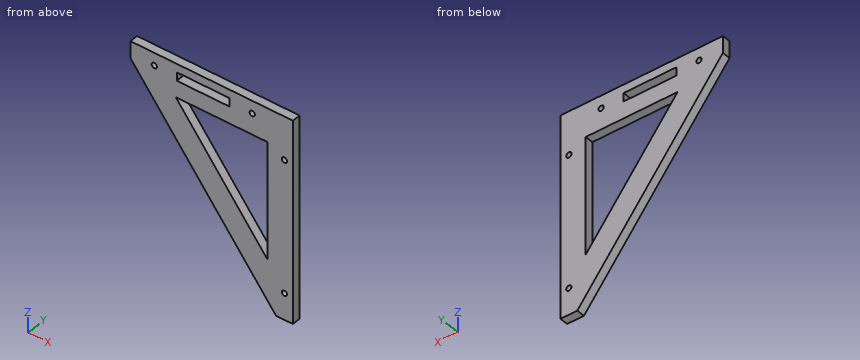
```python
from build123d import *

# Parameters (mm, degrees)
BOSS_EXTRUDE1_DEPTH = 3.175
SKETCH3_W           = 55
SKETCH3_H           = 6.35
BOSS_EXTRUDE3_DEPTH = 3.175
SKETCH5_W           = 6.35
SKETCH5_H           = 76.35
BOSS_EXTRUDE4_DEPTH = 3.175
SKETCH2_R           = 1
SKETCH2_W           = 20
SKETCH2_H           = 3.175
CUT_EXTRUDE1_DEPTH  = 3.175
CUT_EXTRUDE2_DEPTH  = 3.175


with BuildPart() as part:
    # Sketch1 → Boss-Extrude1 (new body)
    with BuildSketch(Plane(origin=(0, 0, 0), x_dir=(1, 0, 0), z_dir=(0, 1, 0))):
        Polygon((0, 0), (55, 0), (55, 70), align=None)
    extrude(amount=BOSS_EXTRUDE1_DEPTH)

    # Sketch3 → Boss-Extrude3 (add)
    with BuildSketch(Plane.XZ):
        with Locations((27.5, 3.175)):
            Rectangle(SKETCH3_W, SKETCH3_H)
    extrude(amount=-BOSS_EXTRUDE3_DEPTH)

    # Sketch5 → Boss-Extrude4 (add)
    with BuildSketch(Plane.XZ):
        with Locations((58.175, -31.825)):
            Rectangle(SKETCH5_W, SKETCH5_H)
    extrude(amount=-BOSS_EXTRUDE4_DEPTH)

    # Sketch2 → Cut-Extrude1 (cut)
    with BuildSketch(Plane(origin=(0, 3.175, 0), x_dir=(1, 0, 0), z_dir=(0, 1, 0))):
        with Locations(Location((9, -1.5875, 0), (0, 0, 270))):
            Circle(SKETCH2_R)
        with Locations(Location((46, -1.5875, 0), (0, 0, 270))):
            Circle(SKETCH2_R)
        with Locations(Location((58.175, 60, 0), (0, 0, 270))):
            Circle(SKETCH2_R)
        with Locations(Location((58.175, 10, 0), (0, 0, 270))):
            Circle(SKETCH2_R)
        with Locations((27.5, -1.5875)):
            Rectangle(SKETCH2_W, SKETCH2_H)
    extrude(amount=-CUT_EXTRUDE1_DEPTH, mode=Mode.SUBTRACT)

    # Sketch6 → Cut-Extrude2 (cut)
    with BuildSketch(Plane(origin=(0, 3.175, 0), x_dir=(1, 0, 0), z_dir=(0, 1, 0))):
        Polygon((51.825, 6.35), (17.102700256, 6.35), (51.825, 50.542017856), align=None)
    extrude(amount=-CUT_EXTRUDE2_DEPTH, mode=Mode.SUBTRACT)


solid = part.part
```
Verification items for the finished model (mm, model axes). Coordinates: 2 decimals unless noted, no trailing zeros. Write each loop counter-clockwise with the first axis right and the second up, starting at its lowest first coordinate (ties: lowest second). Pieces come first, ordered by that corner, then holes. Notation, with made-up numbers: (-16, 31) - (26, 31) arc R22 ccw to (26, 70) - close; hole circle Ø1 at (76.25, 19.25). An arc over 180 degrees is marked (long way). Write item = value, one per line.
Q1. Material ranges on L1, parallel to Z at x = 20, y = 2.9 (3 decimals); L2, parallel to X at y = 1.3, z = -10 (3 decimals); L3, parallel to Z at x = 45.5, y = 2.05, recorded low to high. Write a range as from..to.
Answer:
L1 = -25.455..-10.037, -6.35..0, 3.175..6.35
L2 = 7.857..19.971, 51.825..57.175, 59.175..61.35
L3 = -57.91..-42.49, -6.35..0.72, 2.45..6.35
Q2. Go/stop test with flat-tipped pins: pin 1 Ø1.6 at (x, z) = (46, 1.59) entering from -Y; pin 2 Ø1 at (y, z) = (1.5, -37.5) entering from -X; pin 3 Ø3 at (x, z) = (58.175, -60) entering from -Y. Record where each tip stops, or that it passes through.
Answer:
pin_1 = through
pin_2 = 29.07
pin_3 = 0
Q3. Cross-section at B-B (x = 46). Give the number of separate pieces and of enclosed holes in the cut face, plus the area to 3 significant figures.
Answer:
separate_pieces = 3
enclosed_holes = 0
area = 82.9 mm²
Q4. Cross-section at A-A (z = -40). Enter the section's corners in (x, y) (3 decimals), plus the area to 3 significant figures.
Answer:
outline = (31.429, 0) - (43.542, 0) - (43.542, 3.175) - (31.429, 3.175) - close; (51.825, 0) - (61.35, 0) - (61.35, 3.175) - (51.825, 3.175) - close
area = 68.7 mm²
